Autodesk Inventor part; units mm, degrees
ref_plane "YZ Plane" through (0, 0, 0) normal (1, 0, 0) x (0, 1, 0)
ref_plane "XZ Plane" through (0, 0, 0) normal (0, 1, 0) x (-1, 0, 0)
ref_plane "XY Plane" through (0, 0, 0) normal (0, 0, 1) x (1, 0, 0)
sketch "Esquisse1" plane through (0, 0, 0) normal (0, 0, 1) x (1, 0, 0)
  line L0 (-30, -30) -> (30, -30)
  line L1 (30, -30) -> (30, 30)
  line L2 (30, 30) -> (-30, 30)
  line L3 (-30, 30) -> (-30, -30)
  line L4 (-30, -30) -> (30, 30) construction
  line L5 (30, -30) -> (-30, 30) construction
  point P0 (0, 0)
  dimension "d0" = 60
  dimension "d1" = 60
extrude "Extrusion1" add sketch "Esquisse1" along normal mid plane 11
sketch "Esquisse2" plane through (0, 0, 5.5) normal (0, 0, 1) x (1, 0, 0)
  point P0 (0, 0)
  point P1 (-25, 25)
  point P2 (25, 25)
  point P3 (25, -25)
  point P4 (-25, -25)
  dimension "d4" = 50
  dimension "d5" = 50
  dimension "d7" = 25
  dimension "d8" = 25
hole "Perçage1" at (-25, 25, 5.5) at (25, 25, 5.5) at (25, -25, 5.5) at (-25, -25, 5.5) direction (0, 0, -1) diameter 4.4 end through all counterbore diameter 6.45 counterbore depth 3.16
fillet "Congé1" radius 2 4 edges at (-30, 30, 0) (30, 30, 0) (30, -30, 0) (-30, -30, 0)
sketch "Esquisse3" plane through (-28, -30, -5.5) normal (0, -1, 0) x (1, 0, 0)
  line L0 (56, 0) -> (0, 0)
  point P0 (28, 5.5)
  point P1 (5, 3)
  point P2 (8, 3)
  dimension "d17" = 3
  dimension "d18" = 3
  dimension "d19" = 5
equation "\"pi\" = 3.141593"
equation "\"nombredor\" = 1.61803"
properties part number "Ventillateur_60x60x11" material "Plastique ABS"
Model file for the job. Use its own axes, mm. A direction names the side the tool comes from. Round coordinates to 2 decimals unless told otherwise and drop trailing zeros. Order: outer loops, then holes, each group sorted by start corner. A loop starts at its lowest first (then second) coordinate and runs counter-clockwise, first axis right, second up. Notation, with made-up numbers: M 39.5,-38 L 72.5,-38 A9 cw 72.5,-33 Z; hole C 19.5,-19.5 d10. An arc over 180 degrees is marked long. Write each question's results on one line, items separated by ' | '. Start each with the question number.
(1) Which spindle directions (+Z, -Z, +X, -X, +Y, -Y) get a long thin tool onto all of the face, cutting with end or side? Do faces 5 (the face through (0, -30, 0)), 6 (the face through (27.1, -26.4, 2.34)). Say none if no direction does.
(2) Saw through at A-A, the plane y = -25. Give the cut face in (x, z) (3 decimals).
(3) Saw through at B-B, the plane z = 4.75. Give the cut face in (x, y) (3 decimals), then the cut area to 3 significant figures.
(4) Drop flat-ended pins along their axis: pin 1 (7.5 mm diameter, centred on x = 25, y = -25, fed in from +Z); pin 2 (3 mm diameter, centred on x = 26, y = 25.5, fed in from +Z). Give the stop position or say it passes through.
(5) Two-plate mould, pull along X, no slides. Class faces 1 (the face through (27.148, 25.477, -1.635)), 2 (the face through (29.4, 29.43, -0.08)), 3 (the face through (0, 0, -5.5)), 4 (the face through (-22.9, -26.4, 2.34)): pulls with the +X half, pulls with the -X half, needs draft (parallel to the pull), parting line crosses it, or undercut.
(6) Probe probe 1 along X at (y, z) = (-25, 0.5); probe 2 along X at (y, z) = (25, 3.9) (3 decimals). List the from-to ranges inside material, lowest first. Write a range as from..to.
(7) Saw through at D-D, the plane z = -3. Give the cut face in (x, y).
Established:
1) face 5: +Z, -Z, +X, -X, -Y | face 6: +Z
2) outline: M -30,-5.5 L -27.2,-5.5 L -27.2,2.34 L -28.225,2.34 L -28.225,5.5 L -30,5.5 Z; M -22.8,-5.5 L 22.8,-5.5 L 22.8,2.34 L 21.775,2.34 L 21.775,5.5 L -21.775,5.5 L -21.775,2.34 L -22.8,2.34 Z; M 27.2,-5.5 L 30,-5.5 L 30,5.5 L 28.225,5.5 L 28.225,2.34 L 27.2,2.34 Z
3) outline: M -30,-28 A2 ccw -28,-30 L 28,-30 A2 ccw 30,-28 L 30,28 A2 ccw 28,30 L -28,30 A2 ccw -30,28 Z; hole C -25,-25 d6.45; hole C -25,25 d6.45; hole C 25,-25 d6.45; hole C 25,25 d6.45 | area: 3,470 mm^2
4) pin 1: stops at z = 5.5 | pin 2: stops at z = 2.34
5) face 1: undercut | face 2: pulls with the +X half | face 3: needs draft | face 4: undercut
6) probe 1: x = -30..-27.2, -22.8..22.8, 27.2..30 | probe 2: x = -30..-28.225, -21.775..21.775, 28.225..30
7) outline: M -30,-28 A2 ccw -28,-30 L 28,-30 A2 ccw 30,-28 L 30,28 A2 ccw 28,30 L -28,30 A2 ccw -30,28 Z; hole C -25,-25 d4.4; hole C -25,25 d4.4; hole C 25,-25 d4.4; hole C 25,25 d4.4
